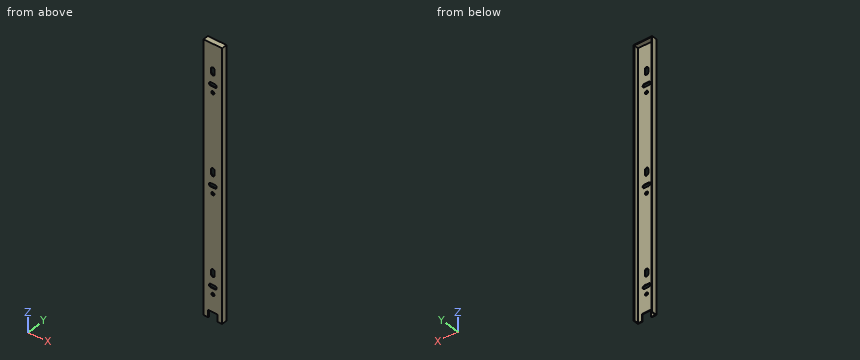
from build123d import *

# Parameters (mm, degrees)
EXTRUDE_1_DEPTH     = 350
SKETCH_2_R          = 2
SKETCH_2_W          = 12
SKETCH_2_H          = 9.239849372
CUT_EXTRUDE_1_DEPTH = 3500
SKETCH_3_W          = 22
SKETCH_3_H          = 1
EXTRUDE_2_DEPTH     = 6


with BuildPart() as part:
    # 草图1 → 凸台-拉伸1 (new body)
    with BuildSketch(Plane.XY):
        Polygon((-12, 3.5), (-11, 3.5), (-11, -2.5), (11, -2.5), (11, 3.5), (12, 3.5), (12, -3.5), (-12, -3.5), align=None)
    extrude(amount=EXTRUDE_1_DEPTH)

    # 草图2 → 切除-拉伸1 (cut)
    with BuildSketch(Plane.XZ.offset(3.5)):
        with Locations((0, 287.75)):
            Circle(SKETCH_2_R)
        with Locations((0, 159.75)):
            Circle(SKETCH_2_R)
        with Locations((0, 31.75)):
            Circle(SKETCH_2_R)
        with BuildLine():
            Line((-2.75, 300), (2.75, 300))
            ThreePointArc((2.75, 300), (5, 297.75), (2.75, 295.5))
            Line((2.75, 295.5), (-2.75, 295.5))
            ThreePointArc((-2.75, 295.5), (-5, 297.75), (-2.75, 300))
        make_face()
        with BuildLine():
            Line((-2.25, 317.75), (-2.25, 312.25))
            ThreePointArc((-2.25, 312.25), (0, 310), (2.25, 312.25))
            Line((2.25, 312.25), (2.25, 317.75))
            ThreePointArc((2.25, 317.75), (0, 320), (-2.25, 317.75))
        make_face()
        with BuildLine():
            Line((-2.25, 189.75), (-2.25, 184.25))
            ThreePointArc((-2.25, 184.25), (0, 182), (2.25, 184.25))
            Line((2.25, 184.25), (2.25, 189.75))
            ThreePointArc((2.25, 189.75), (0, 192), (-2.25, 189.75))
        make_face()
        with BuildLine():
            Line((2.75, 167.5), (-2.75, 167.5))
            ThreePointArc((-2.75, 167.5), (-5, 169.75), (-2.75, 172))
            Line((-2.75, 172), (2.75, 172))
            ThreePointArc((2.75, 172), (5, 169.75), (2.75, 167.5))
        make_face()
        with BuildLine():
            Line((-2.25, 61.75), (-2.25, 56.25))
            ThreePointArc((-2.25, 56.25), (0, 54), (2.25, 56.25))
            Line((2.25, 56.25), (2.25, 61.75))
            ThreePointArc((2.25, 61.75), (0, 64), (-2.25, 61.75))
        make_face()
        with BuildLine():
            Line((2.75, 39.5), (-2.75, 39.5))
            ThreePointArc((-2.75, 39.5), (-5, 41.75), (-2.75, 44))
            Line((-2.75, 44), (2.75, 44))
            ThreePointArc((2.75, 44), (5, 41.75), (2.75, 39.5))
        make_face()
        with Locations((0, 4.619924686)):
            Rectangle(SKETCH_2_W, SKETCH_2_H)
    extrude(amount=-CUT_EXTRUDE_1_DEPTH, mode=Mode.SUBTRACT)

    # 草图3 → 凸台-拉伸2 (add)
    with BuildSketch(Plane(origin=(0, -2.5, 0), x_dir=(1, 0, 0), z_dir=(0, 1, 0))):
        with Locations((0, -349.5)):
            Rectangle(SKETCH_3_W, SKETCH_3_H)
    extrude(amount=EXTRUDE_2_DEPTH)


solid = part.part
Can you work these out from the model? Positions are in its coordinate system, mm. Round coordinates to 2 decimals unless told otherwise and drop trailing zeros. Write each loop counter-clockwise with the first axis right and the second up, starting at its lowest first coordinate (ties: lowest second). Pieces come first, ordered by that corner, then holes. Notation, with made-up numbers: (55, 65) - (110, 65) arc R17 cw to (110, 87) - close; hole circle Ø10 at (61, -4). An arc over 180 degrees is marked (long way). Write each question's results on one line, items separated by ' | '. Start each with the question number.
1) Please list where these lines run through material, in increasing order: line 1 (X direction, y = 0.25, z = 118); line 2 (X direction, y = -3.15, z = 287.75); line 3 (Y direction, x = 7, z = 210.5).
2) Suppose I cut it at B-B (y = 1.5). List the corners of the cut face in (x, z) for me.
3) Suppose I cut it at A-A (z = 266.5). List the corners of the cut face in (x, y) for me.
4) For pin 1 Ø4 at (x, y) = (6, 1.5) entering from -Z; pin 2 Ø3 at (x, z) = (0, 287.75) entering from +Y; pin 3 Ø6.5 at (x, z) = (1.5, 191) entering from +Y; pin 4 Ø1.1 at (x, y) = (0.5, -3) entering from -Z, each with a flat end and sliding along its axis, tell me the tip position at first contact or that it passes through.
Here are the results:
1) line 1: x = -12 to -11, 11 to 12 | line 2: x = -12 to -2, 2 to 12 | line 3: y = -3.5 to -2.5
2) outline: (-12, 0) - (-11, 0) - (-11, 349) - (11, 349) - (11, 0) - (12, 0) - (12, 350) - (-12, 350) - close
3) outline: (-12, -3.5) - (12, -3.5) - (12, 3.5) - (11, 3.5) - (11, -2.5) - (-11, -2.5) - (-11, 3.5) - (-12, 3.5) - close
4) pin 1: stops at z = 349 | pin 2: passes through | pin 3: stops at y = -2.5 | pin 4: stops at z = 9.24
